Build history of the part. All positions in model axes, mm. Face numbers are marked on the shaded views. A direction names the side the tool comes from. Coordinates: 2 decimals unless noted, no trailing zeros. Loops run counter-clockwise (first coordinate to the right, second up) from the corner with the lowest first, then second, coordinate; pieces in that order, holes last.
(1) Slice it at B-B (y = 6.75). Give the cut face in (x, z) (3 decimals), and give its area (3 significant figures).
(2) Wall check: L1, parallel to X at y = 3.25, z = -0.1 (3 decimals); L2, parallel to Y at x = 5.75, z = -0.7; L3, parallel to Z at x = -4.5, y = 6.5. Give the ranges that are in metal, low to high.
(3) Slice it at C-C (x = -5). Give the cut face in (y, z).
(4) Slice it at A-A (y = 3.81). Give the cut face in (x, z) (3 decimals), and give its area (3 significant figures).
(5) Two-plate mould, pull along X, no slides. Class the marked faces 4, 5 and 6: pulls with the +X half, pulls with the -X half, needs draft (parallel to the pull), parting line crosses it, or undercut.
(6) Slice it at D-D (z = -0.5). Give the cut face in (x, y) (3 decimals), and give its area (3 significant figures).
(7) Tool access for the marked faces 1, 2 and 3: list every direction of +Z, -Z, +X, -X, +Y, -Y with a clear straight run to the whole face (end or side of a thin tool).
(8) Flat gauge pin, fed straight in: P1, Ø3, axis at x = -8, y = 3, coming from the +Z side. Where does the tip first touch, or does it go through?
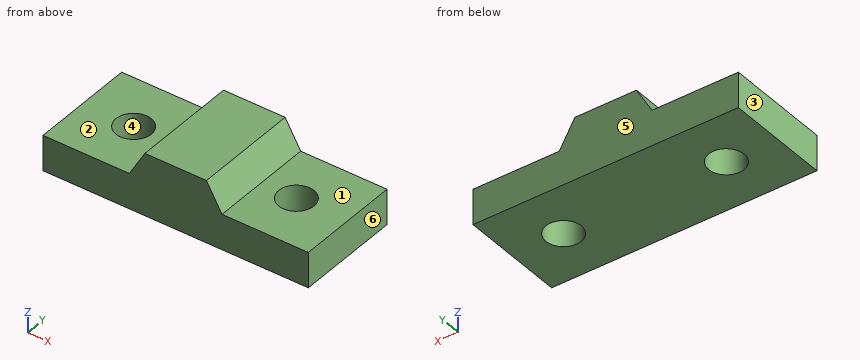
from build123d import *

# Parameters (mm, degrees)
SKETCH1_W           = 6.1976
SKETCH1_H           = 2.54
BOSS_EXTRUDE1_DEPTH = 7.62
CUT_EXTRUDE2_REACH  = 14.993
SKETCH3_R           = 1.27


with BuildPart() as part:
    # Sketch1 → Boss-Extrude1 (new body)
    with BuildSketch(Plane(origin=(0, 0, 0), x_dir=(1, 0, 0), z_dir=(0, 1, 0))):
        Polygon((0, -3.205739983), (0, -1.27), (-3.3274, -1.27), (-2.2098, -3.205739983), align=None)
        Polygon((3.3274, -1.27), (0, -1.27), (0, -3.205739983), (2.2098, -3.205739983), align=None)
        with Locations((6.4262, 0)):
            Rectangle(SKETCH1_W, SKETCH1_H)
        Polygon((-3.3274, -1.27), (0, -1.27), (3.3274, -1.27), (3.3274, 1.27), (-3.3274, 1.27), align=None)
        with Locations((-6.4262, 0)):
            Rectangle(SKETCH1_W, SKETCH1_H)
    extrude(amount=BOSS_EXTRUDE1_DEPTH)

    # Sketch3 → Cut-Extrude2 (cut, up to next)
    with BuildSketch(Plane.XY.offset(3.205739983), mode=Mode.PRIVATE) as cut_extrude2_sk1:
        with Locations((-5.842, 3.81)):
            Circle(SKETCH3_R)
    cut_extrude2_tool1 = extrude(cut_extrude2_sk1.sketch, amount=-CUT_EXTRUDE2_REACH, mode=Mode.PRIVATE) & part.part
    cut_extrude2 = cut_extrude2_tool1.solids().sort_by_distance((-5.842, 3.81, 3.20574))[0]
    add(cut_extrude2, mode=Mode.SUBTRACT)

    # Mirror2: Cut-Extrude2 across plane
    add(cut_extrude2.mirror(Plane(origin=(0, 0, 0), x_dir=(0, 0, 1), z_dir=(1, 0, 0))), mode=Mode.SUBTRACT)


solid = part.part
Response values:
1. outline: (-9.525, -1.27) - (9.525, -1.27) - (9.525, 1.27) - (3.327, 1.27) - (2.21, 3.206) - (-2.21, 3.206) - (-3.327, 1.27) - (-9.525, 1.27) - close
1. area: 59.1 mm2
2. L1: x = -9.525 to -6.982, -4.702 to 4.702, 6.982 to 9.525
2. L2: y = 0 to 2.54, 5.08 to 7.62
2. L3: z = -1.27 to 1.27
3. outline: (0, -1.27) - (2.86, -1.27) - (2.86, 1.27) - (0, 1.27) - close; (4.76, -1.27) - (7.62, -1.27) - (7.62, 1.27) - (4.76, 1.27) - close
4. outline: (-9.525, -1.27) - (-7.112, -1.27) - (-7.112, 1.27) - (-9.525, 1.27) - close; (-4.572, -1.27) - (4.572, -1.27) - (4.572, 1.27) - (3.327, 1.27) - (2.21, 3.206) - (-2.21, 3.206) - (-3.327, 1.27) - (-4.572, 1.27) - close; (7.112, -1.27) - (9.525, -1.27) - (9.525, 1.27) - (7.112, 1.27) - close
4. area: 46.2 mm2
5. face 4: undercut
5. face 5: needs draft
5. face 6: pulls with the +X half
6. outline: (-9.525, 0) - (9.525, 0) - (9.525, 7.62) - (-9.525, 7.62) - close; hole circle Ø2.54 at (-5.842, 3.81); hole circle Ø2.54 at (5.842, 3.81)
6. area: 135 mm2
7. face 1: +Z, +X, +Y, -Y
7. face 2: +Z, -X, +Y, -Y
7. face 3: +Z, -Z, -X, +Y, -Y
8. P1: stops at z = 1.27
